from build123d import *

# Parameters (mm, degrees)
SKETCH2_R          = 1.5
CUT_EXTRUDE1_DEPTH = 9.25


with BuildPart() as part:
    # Sketch1 → Revolve1 (revolve)
    with BuildSketch(Plane(origin=(0, 0, 0), x_dir=(1, 0, 0), z_dir=(0, 1, 0))):
        with BuildLine():
            Line((-4.125, 0), (4.125, 0))
            Line((4.125, 0), (4.125, 2.6))
            Line((4.125, 2.6), (2.333030278, 1.7))
            Line((2.333030278, 1.7), (1.833030278, 1.7))
            ThreePointArc((1.833030278, 1.7), (0, 2.5), (-1.833030278, 1.7))
            Line((-1.833030278, 1.7), (-2.333030278, 1.7))
            Line((-2.333030278, 1.7), (-4.125, 2.6))
            Line((-4.125, 2.6), (-4.125, 0))
        make_face()
    revolve(axis=Axis((-4.125, 0, 0), (1, 0, 0)))

    # Sketch2 → Cut-Extrude1 (cut, through all)
    with BuildSketch(Plane(origin=(4.125, 0, 0), x_dir=(0, 0, -1), z_dir=(1, 0, 0))):
        Circle(SKETCH2_R)
    extrude(amount=-CUT_EXTRUDE1_DEPTH, mode=Mode.SUBTRACT)


solid = part.part
Design review of the part built by this model. Coordinates are the model's own, in mm. A direction names the side the tool comes from. Round coordinates to 2 decimals unless told otherwise and drop trailing zeros. Write each loop counter-clockwise with the first axis right and the second up, starting at its lowest first coordinate (ties: lowest second). Pieces come first, ordered by that corner, then holes. Notation, with made-up numbers: M 27.25,-30 L 66.25,-30 A28 cw 66.25,8 Z; hole C -14.5,22.25 d4. An arc over 180 degrees is marked long. One line per item, written item: value. Start each with the question number.
1. Take a section at A-A on z = 0. State the section outline as (x, y) points (3 decimals), then the cut area to 3 significant figures.
2. To check wall thickness, follow probe 1 along X at (y, z) = (-0.7, -2.1) (3 decimals); probe 2 along X at (y, z) = (0.8, -1.8) (3 decimals); probe 3 along Y at (x, z) = (2, 1.35). State the ranges of each line that lie inside material, in increasing order. Write a range as from..to.
3. Clearance check with a flat-ended pin moving along its axis: P1, Ø1, axis at x = 1.5, y = 0, coming from the -Z side. State where the tip first meets the part, or that it passes through.
4. Take a section at C-C on x = 2. State the section outline as (y, z) points, then the cut area to 3 significant figures.
5. Draft analysis for pull direction X (two halves, no side actions). For faces 1 (the face through (4.125, 0, 2)), 2 (the face through (2.08, -1.66, 0.37)), 3 (the face through (0.06, 0.07, 1.5)), state which applies: pulls with the +X half, pulls with the -X half, needs draft (parallel to the pull), parting line crosses it, or undercut.
6. For faces 4 (the face through (-2.09, -1.66, 0.37)), 5 (the face through (-4.125, 0, -2)), list the 3-axis set-ups (+Z, -Z, +X, -X, +Y, -Y) from which the entire face can be reached by the end or side of a thin tool; tool diameter is ignored.
7. Take a section at D-D on y = 2.15. State how many separate pieces and enclosed holes the cut face has, then the cut area to 3 significant figures.
Computed:
1. outline: M -4.125,-2.6 L -2.333,-1.7 L -1.833,-1.7 A2.5 ccw 1.833,-1.7 L 2.333,-1.7 L 4.125,-2.6 L 4.125,-1.5 L -4.125,-1.5 Z; M -4.125,1.5 L 4.125,1.5 L 4.125,2.6 L 2.333,1.7 L 1.833,1.7 A2.5 ccw -1.833,1.7 L -2.333,1.7 L -4.125,2.6 Z
1. area: 10.6 mm²
2. probe 1: x = -4.125..-3.356, -1.162..1.162, 3.356..4.125
2. probe 2: x = -4.125..-2.87, -1.539..1.539, 2.87..4.125
2. probe 3: y = -1.03..-0.65, 0.65..1.03
3. P1: stops at z = -2.29
4. outline: C 0,0 d3.4; hole C 0,0 d3
4. area: 2.01 mm²
5. face 1: pulls with the +X half
5. face 2: undercut
5. face 3: needs draft
6. face 4: none
6. face 5: +Z, -Z, -X, +Y, -Y
7. separate pieces: 3
7. enclosed holes: 0
7. area: 8.54 mm²
